```python
from build123d import *

# Parameters (mm, degrees)
ESQUISSE1_R             = 9.9
BOSS_EXTRU_1_DEPTH      = 15
ENL_V_MAT_EXTRU_1_DEPTH = 2
ESQUISSE6_R             = 9.9
ENL_V_MAT_EXTRU_2_DEPTH = 10
ESQUISSE8_R             = 12
BOSS_EXTRU_2_DEPTH      = 8


with BuildPart() as part:
    # Esquisse1 → Boss.-Extru.1 (new body)
    with BuildSketch(Plane.XY):
        Circle(ESQUISSE1_R)
    extrude(amount=BOSS_EXTRU_1_DEPTH)

    # Esquisse4 → Enlèv. mat.-Extru.1 (cut)
    # profile 1 of 2: a face of its own
    with BuildSketch(Plane.XY.offset(15)):
        Polygon((0.186527371, 4.159848226), (-6.163470089, 4.159848226), (-6.444587129, 4.159848226), (-7.287953489, 3.696780826), (-7.750975169, 2.853399226), (-7.750975169, 2.572297426), (-7.750975169, -0.602651774), (-7.750975169, -0.879638774), (-7.287953489, -1.723020374), (-6.444587129, -2.190179714), (-6.163470089, -2.190179714), (-5.369725169, -2.190179714), (-5.369725169, -5.365174634), (-5.369725169, -5.501610734), (-5.138214329, -5.923278674), (-4.716531149, -6.158927174), (-4.575972629, -6.158927174), (-2.988475169, -6.158927174), (-2.852039069, -6.158927174), (-2.430371129, -5.923278674), (-2.194722629, -5.501610734), (-2.194722629, -5.365174634), (-2.194722629, -2.190179714), (0.186527371, -2.190179714), (4.155251971, -5.365174634), (4.155251971, 7.334797426), align=None)
        Polygon((2.567777371, -1.871854214), (0.980302771, -0.602651774), (-6.163470089, -0.602651774), (-6.163470089, 2.572297426), (0.980302771, 2.572297426), (2.567777371, 3.841484626), align=None, mode=Mode.SUBTRACT)
    # profile 2 of 2: a face of its own
    with BuildSketch(Plane.XY.offset(15)):
        Polygon((7.727126971, 0.984822826), (7.727126971, 0.517640626), (7.193879371, -0.887944574), (6.048745771, -2.041345874), (5.742802771, -2.190179714), (5.742802771, 4.159848226), (6.044630971, 4.011029626), (7.189764571, 2.857514026), (7.727126971, 1.456119826), align=None)
    extrude(amount=-ENL_V_MAT_EXTRU_1_DEPTH, mode=Mode.SUBTRACT)

    # Esquisse6 → Enlèv. mat.-Extru.2 (cut)
    with BuildSketch(Plane(origin=(0, 0, 0), x_dir=(-1, 0, 0), z_dir=(0, 0, -1))):
        Circle(ESQUISSE6_R)
    extrude(amount=-ENL_V_MAT_EXTRU_2_DEPTH, mode=Mode.SUBTRACT)

    # Esquisse8 → Boss.-Extru.2 (add)
    with BuildSketch(Plane(origin=(0, 0, 10), x_dir=(-1, 0, 0), z_dir=(0, 0, -1))):
        Circle(ESQUISSE8_R)
    extrude(amount=BOSS_EXTRU_2_DEPTH)


solid = part.part
```
Geometry check sheet. Reference: the model listing, model coordinates, mm. Coordinates: 2 decimals unless noted, no trailing zeros. Write each loop counter-clockwise with the first axis right and the second up, starting at its lowest first coordinate (ties: lowest second). Pieces come first, ordered by that corner, then holes. Notation, with made-up numbers: M 2.25,42 L 41.25,42 A30 ccw 41.25,73 Z; hole C 46.25,-13 d8. An arc over 180 degrees is marked long. Answer as a JSON object with one key per item and string values.
1. Go/stop test with flat-tipped pins: pin 1 Ø3 at (y, z) = (-8.5, 5) entering from +X; pin 2 Ø2 at (y, z) = (0, 14.5) entering from +X; pin 3 Ø1 at (x, z) = (-3.5, 13.5) entering from -Y. Record where each tip stops, or that it passes through.
Answers below:
{"pin 1": "stops at x = 9.75", "pin 2": "stops at x = 9.9", "pin 3": "stops at y = -9.43"}
2. Draft check along X on faces 1 (the flat face through (0, -4, 15)), 2 (the flat face through (1.763, 3.198, 14.014)), 3 (the cylindrical face through (11.99, 0.53, 6.06)). Enter one of: released by +X, released by -X, zero draft, split by the parting line, or undercut.
Answers below:
{"face 1": "zero draft", "face 2": "undercut", "face 3": "split by the parting line"}
3. Section check B-B, the plane y = 6.5. Enter the section's corners in (x, z).
Answers below:
{"outline": "M -10.09,2 L 10.09,2 L 10.09,10 L 7.47,10 L 7.47,15 L 4.16,15 L 4.16,13 L 3.11,13 L 3.11,15 L -7.47,15 L -7.47,10 L -10.09,10 Z"}
4. Section check A-A, the plane x = -1. Enter the section's corners in (y, z).
Answers below:
{"outline": "M -11.96,2 L 11.96,2 L 11.96,10 L 9.85,10 L 9.85,15 L 4.16,15 L 4.16,13 L 2.57,13 L 2.57,15 L -0.6,15 L -0.6,13 L -2.19,13 L -2.19,15 L -9.85,15 L -9.85,10 L -11.96,10 Z"}
5. Scan lines: L1, parallel to X at y = -4, z = 14.25; L2, parallel to Z at x = -5.75, y = -9.5; L3, parallel to X at y = 5.5, z = 13.5. Record each from-to range of solid material in increasing order.
Answers below:
{"L1": "x = -9.06 to -5.37, -2.19 to 2.45, 4.16 to 9.06", "L2": "z = 2 to 10", "L3": "x = -8.23 to 1.86, 4.16 to 8.23"}
6. Section check C-C, the plane z = 7.5. Enter the section's corners in (x, y), plus the area to 3 significant figures.
Answers below:
{"outline": "C 0,0 d24", "area": "452 mm²"}
7. Section check D-D, the plane x = -6.75. Enter the section's corners in (y, z), plus the area to 3 significant figures.
Answers below:
{"outline": "M -9.92,2 L 9.92,2 L 9.92,10 L 7.24,10 L 7.24,15 L 3.99,15 L 3.99,13 L -2.02,13 L -2.02,15 L -7.24,15 L -7.24,10 L -9.92,10 Z", "area": "219 mm²"}
